Read the model definition and answer for the solid it produces. Units are mm, in the model's axes. A direction names the side the tool comes from. Coordinates: 2 decimals unless noted, no trailing zeros. Order: outer loops, then holes, each group sorted by start corner. A loop starts at its lowest first (then second) coordinate and runs counter-clockwise, first axis right, second up. Notation, with made-up numbers: (74.5, 87) -> (108.5, 87) arc R20 ccw to (108.5, 110) -> close; hole circle Ø10 at (28.25, 29.25). An arc over 180 degrees is marked (long way). Answer as a JSON object with one key per item and string values. Group by question number.
1) Consider L1, parallel to X at y = 1.2, z = -53.6; L2, parallel to X at y = 3.4, z = -53.6; L3, parallel to X at y = 10, z = -51.5. Determine where each line is inside the solid, lowest interval first.
2) A tool of negligible diameter and unlimited length cuts with its end or side. For faces 1 (the flat face through (0, 10, -29)), 2 (the flat face through (27.3, 10, -29)), 3 (the cylindrical face through (13.369, 1.703, -28.89)), 4 (the flat face through (14, 7.25, -57)), from which of +Z, -Z, +X, -X, +Y, -Y can it reach the whole face along a straight path? Write none if from no direction.
3) Section C-C on y = 6 is taken. Determine the outline of the cut face in (x, z).
4) Determine the mould class of faces 5 (the flat face through (13, 4, -58.6)), 6 (the cylindrical face through (33.65, 2.46, -4.14)), 7 (the flat face through (-10, 2, -29)) for opening direction X: released by +X, released by -X, zero draft, split by the parting line, or undercut.
5) Given pin 1 (2 mm diameter, centred on x = 14, z = -1, fed in from +Y); pin 2 (5 mm diameter, centred on x = -5, z = -53.6, fed in from +Y); pin 3 (2.5 mm diameter, centred on x = 14.5, z = -57, fed in from +Y); pin 4 (4.5 mm diameter, centred on x = 10.5, y = 3.5, fed in from +Z), each flat-ended and moving along its own axis, determine where each tip first touches the part or whether it passes through.
6) Section A-A on z = -53.6 is taken. Determine the outline of the cut face in (x, y), and give its area (3 significant figures).
7) Section B-B on x = -5 is taken. Determine the outline of the cut face in (y, z).
8) Section D-D on z = -16 is taken. Determine the outline of the cut face in (x, y), and give its area (3 significant figures).
from build123d import *

# Parameters (mm, degrees)
SKETCH_1_W          = 27.3
SKETCH_1_H          = 58.6
EXTRUDE_1_DEPTH     = 14.5
SKETCH_3_R          = 12.8
CUT_EXTRUDE_1_DEPTH = 67.253301805
SKETCH_7_W          = 27.3
SKETCH_7_H          = 7.25
EXTRUDE_2_DEPTH     = 3
EXTRUDE_START       = -58.6
EXTRUDE_3_DEPTH     = 2.5
SKETCH_1_3_W        = 10
SKETCH_1_3_H        = 58.6
SKETCH_1_3_R        = 1.6
EXTRUDE_4_DEPTH     = 5


with BuildPart() as part:
    # Sketch 1 → Extrude 1 (new body)
    with BuildSketch(Plane(origin=(0, 0, 0), x_dir=(1, 0, 0), z_dir=(0, 1, 0))):
        with Locations((13.65, 29.3)):
            Rectangle(SKETCH_1_W, SKETCH_1_H)
    extrude(amount=EXTRUDE_1_DEPTH)

    # Sketch 3 → Cut-Extrude 1 (cut, through all)
    with BuildSketch(Plane.XY):
        with Locations((13.65, 14.5)):
            Circle(SKETCH_3_R)
    extrude(amount=-CUT_EXTRUDE_1_DEPTH, mode=Mode.SUBTRACT)

    # Sketch 7 → Extrude 2 (add)
    with BuildSketch(Plane(origin=(0, 0, -58.6), x_dir=(-1, 0, 0), z_dir=(0, 0, -1))):
        with Locations((-13.65, 3.625)):
            Rectangle(SKETCH_7_W, SKETCH_7_H)
    extrude(amount=-EXTRUDE_2_DEPTH)

    # Sketch 7_2 → Extrude 3 (add)
    with BuildSketch(Plane(origin=(0, 0, -58.6), x_dir=(-1, 0, 0), z_dir=(0, 0, -1)).offset(EXTRUDE_START)):
        with BuildLine():
            Line((-27.3, 14.5), (-27.3, 7.25))
            Line((-27.3, 7.25), (-24.198815099, 7.25))
            ThreePointArc((-24.198815099, 7.25), (-25.874255259, 10.704267743), (-26.45, 14.5))
            Line((-26.45, 14.5), (-27.3, 14.5))
        make_face()
        with BuildLine():
            Line((-24.198815099, 7.25), (-27.3, 7.25))
            Line((-27.3, 7.25), (-27.3, 0))
            Line((-27.3, 0), (0, 0))
            Line((0, 0), (0, 7.25))
            Line((0, 7.25), (-3.101184901, 7.25))
            ThreePointArc((-3.101184901, 7.25), (-13.65, 1.7), (-24.198815099, 7.25))
        make_face()
        with BuildLine():
            Line((-3.101184901, 7.25), (-24.198815099, 7.25))
            ThreePointArc((-24.198815099, 7.25), (-13.65, 1.7), (-3.101184901, 7.25))
        make_face()
        with BuildLine():
            ThreePointArc((-0.85, 14.5), (-1.425744741, 10.704267743), (-3.101184901, 7.25))
            Line((-3.101184901, 7.25), (0, 7.25))
            Line((0, 7.25), (0, 14.5))
            Line((0, 14.5), (-0.85, 14.5))
        make_face()
    extrude(amount=EXTRUDE_3_DEPTH)

    # Sketch 1_3 → Extrude 4 (add)
    # profile 1 of 2: a face of its own
    with BuildSketch(Plane(origin=(0, 0, 0), x_dir=(1, 0, 0), z_dir=(0, 1, 0))):
        with Locations((32.3, 29.3)):
            Rectangle(SKETCH_1_3_W, SKETCH_1_3_H)
        with Locations(Location((32.3, 53.6, 0), (0, 0, 270))):
            Circle(SKETCH_1_3_R, mode=Mode.SUBTRACT)
        with Locations(Location((32.3, 5, 0), (0, 0, 270))):
            Circle(SKETCH_1_3_R, mode=Mode.SUBTRACT)
    # profile 2 of 2: a face of its own
    with BuildSketch(Plane(origin=(0, 0, 0), x_dir=(1, 0, 0), z_dir=(0, 1, 0))):
        with Locations((-5, 29.3)):
            Rectangle(SKETCH_1_3_W, SKETCH_1_3_H)
        with Locations(Location((-5, 5, 0), (0, 0, 270))):
            Circle(SKETCH_1_3_R, mode=Mode.SUBTRACT)
        with Locations(Location((-5, 53.6, 0), (0, 0, 270))):
            Circle(SKETCH_1_3_R, mode=Mode.SUBTRACT)
    extrude(amount=EXTRUDE_4_DEPTH)


solid = part.part
Worked answers:
{
 "1": {"L1": "x = -10 to -6.6, -3.4 to 30.7, 33.9 to 37.3", "L2": "x = -10 to -6.6, -3.4 to 7.28, 20.02 to 30.7, 33.9 to 37.3", "L3": "x = 0 to 1.67, 25.63 to 27.3"},
 "2": {"face 1": "+Z, -Z, -X, +Y", "face 2": "+Z, -Z, +X, +Y", "face 3": "+Y", "face 4": "+Z, -Z, +Y"},
 "3": {"outline": "(0, -58.6) -> (27.3, -58.6) -> (27.3, 0) -> (0, 0) -> close; hole (4.08, -55.6) -> (23.22, -55.6) -> (23.22, -2.5) -> (4.08, -2.5) -> close"},
 "4": {"face 5": "zero draft", "face 6": "undercut", "face 7": "released by -X"},
 "5": {"pin 1": "stops at y = 7.25", "pin 2": "stops at y = 5", "pin 3": "stops at y = 7.25", "pin 4": "stops at z = 0"},
 "6": {"outline": "(-10, 0) -> (-6.6, 0) -> (-6.6, 5) -> (-10, 5) -> close; (-3.4, 0) -> (30.7, 0) -> (30.7, 5) -> (27.3, 5) -> (27.3, 14.5) -> (26.45, 14.5) arc R12.8 cw to (0.85, 14.5) -> (0, 14.5) -> (0, 5) -> (-3.4, 5) -> close; (33.9, 0) -> (37.3, 0) -> (37.3, 5) -> (33.9, 5) -> close", "area": "206 mm²"},
 "7": {"outline": "(0, -58.6) -> (5, -58.6) -> (5, -55.2) -> (0, -55.2) -> close; (0, -52) -> (5, -52) -> (5, -6.6) -> (0, -6.6) -> close; (0, -3.4) -> (5, -3.4) -> (5, 0) -> (0, 0) -> close"},
 "8": {"outline": "(-10, 0) -> (37.3, 0) -> (37.3, 5) -> (27.3, 5) -> (27.3, 14.5) -> (26.45, 14.5) arc R12.8 cw to (0.85, 14.5) -> (0, 14.5) -> (0, 5) -> (-10, 5) -> close", "area": "238 mm²"}
}
